The listing builds one solid part. Answer for the finished solid, in the listing's coordinates (mm). Face numbers are marked on the shaded views. A direction names the side the tool comes from. Round coordinates to 2 decimals unless told otherwise and drop trailing zeros. Write each loop counter-clockwise with the first axis right and the second up, starting at its lowest first coordinate (ties: lowest second). Pieces come first, ordered by that corner, then holes. Notation, with made-up numbers: (33.5, -35.5) - (63.5, -35.5) arc R30 ccw to (63.5, 3.5) - close; hole circle Ø4 at (2, 79). An arc over 180 degrees is marked (long way). Use a Markdown table: item, result. Add a question column.
1) A cutting plane is placed at B-B (y = 51.5). Give the vertices of the cut face in (x, z).
2) Find the intervals of material crossed by probe 1 along X at (y, z) = (34.55, 22.5); probe 2 along Y at (x, z) = (63.9, 22.25); probe 3 along Y at (x, z) = (16, 24), in increasing order. Write a range as from..to.
3) Determine the mould class of the marked faces 4, 5 and 6 for opening direction Y: +Y half, -Y half, draft (parallel to the pull), parting line (faces both ways), or undercut.
4) A cutting plane is placed at D-D (y = 43). Give the vertices of the cut face in (x, z), then the cut area to 3 significant figures.
5) A tool of negligible diameter and unlimited length cuts with its end or side. For the marked faces 1, 2 and 3, from which of +Z, -Z, +X, -X, +Y, -Y can it reach the whole face along a straight path? Write none if from no direction.
6) A cutting plane is placed at C-C (x = 71.5). Give the vertices of the cut face in (y, z).
7) A cutting plane is placed at A-A (z = 29.5). Give the vertices of the cut face in (x, y), then the cut area to 3 significant figures.
8) Each of these flat-tipped pins is pushed along its axis until it touches: P1, Ø1.5, axis at x = 42, y = 30.5, coming from the +Z side; P2, Ø1.7, axis at y = 23.5, z = 25.5, coming from the -X side; P3, Ø6, axis at y = 32.5, z = 7.5, coming from the -X side; P4, Ø1.6, axis at x = 16, y = 34.5, coming from the +Z side. Where does it stop, or does it pass through?
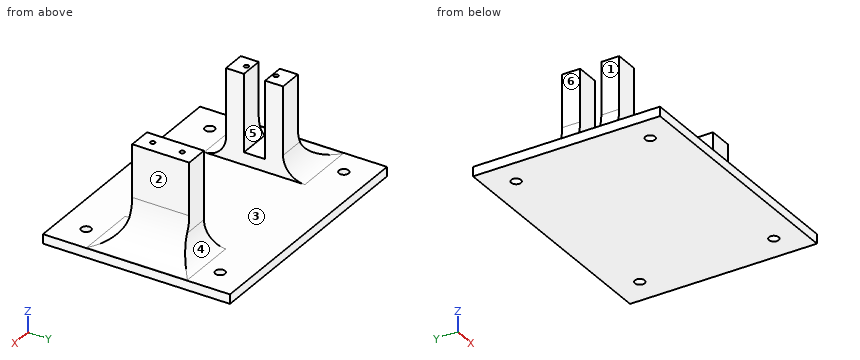
```python
from build123d import *

# Parameters (mm, degrees)
SKETCH078_W     = 80
SKETCH078_H     = 60
PAD029_DEPTH    = 3
SKETCH079_W     = 7.5
SKETCH079_H     = 18.3
PAD030_DEPTH    = 28.8
SKETCH080_R     = 1.55
POCKET038_DEPTH = 5
SKETCH081_R     = 0.75
POCKET039_DEPTH = 15
FILLET024_R     = 12
FILLET025_R     = 7
SKETCH082_W     = 19.5
SKETCH082_H     = 6.8
POCKET040_DEPTH = 24.8


with BuildPart() as part:
    # Sketch078 → Pad029 (new body)
    with BuildSketch(Plane.XY):
        with Locations((40, 30)):
            Rectangle(SKETCH078_W, SKETCH078_H)
    extrude(amount=PAD029_DEPTH)

    # Sketch079 (on Face6 of Pad029) → Pad030 (join)
    with BuildSketch(Plane.XY.offset(3)):
        with Locations((16.1, 30)):
            Rectangle(SKETCH079_W, SKETCH079_H)
        with Locations((63.9, 30)):
            Rectangle(SKETCH079_W, SKETCH079_H)
    extrude(amount=PAD030_DEPTH)

    # Sketch080 (on Face5 of Pad030) → Pocket038 (cut)
    with BuildSketch(Plane.XY.offset(3)):
        with Locations((71.5, 51.5)):
            Circle(SKETCH080_R)
        with Locations((8.5, 51.5)):
            Circle(SKETCH080_R)
        with Locations((71.5, 8.5)):
            Circle(SKETCH080_R)
        with Locations((8.5, 8.5)):
            Circle(SKETCH080_R)
    extrude(amount=-POCKET038_DEPTH, mode=Mode.SUBTRACT)

    # Sketch081 (on Face19 of Pocket038) → Pocket039 (cut)
    with BuildSketch(Plane.XY.offset(31.8)):
        with Locations((16.1, 34.55)):
            Circle(SKETCH081_R)
        with Locations((16.1, 25.05)):
            Circle(SKETCH081_R)
        with Locations((63.9, 34.55)):
            Circle(SKETCH081_R)
        with Locations((63.9, 25.05)):
            Circle(SKETCH081_R)
    extrude(amount=-POCKET039_DEPTH, mode=Mode.SUBTRACT)

    # Fillet024
    fillet024_edges = [part.edges().sort_by_distance(p)[0] for p in [
        (12.35, 30, 3),
        (67.65, 30, 3),
    ]]
    fillet(fillet024_edges, radius=FILLET024_R)

    # Fillet025
    fillet025_edges = [part.edges().sort_by_distance(p)[0] for p in [
        (16.1, 20.85, 3),
        (63.9, 20.85, 3),
        (63.9, 39.15, 3),
        (16.1, 39.15, 3),
    ]]
    fillet(fillet025_edges, radius=FILLET025_R)

    # Sketch082 (on Face19 of Pocket039) → Pocket040 (cut)
    with BuildSketch(Plane.XY.offset(31.8)):
        with Locations((10.1, 30)):
            Rectangle(SKETCH082_W, SKETCH082_H)
    extrude(amount=-POCKET040_DEPTH, mode=Mode.SUBTRACT)


solid = part.part
```
Entries:
| question | item | result |
|---|---|---|
| 1 | outline | (0, 0) - (6.95, 0) - (6.95, 3) - (0, 3) - close; (10.05, 0) - (69.95, 0) - (69.95, 3) - (10.05, 3) - close; (73.05, 0) - (80, 0) - (80, 3) - (73.05, 3) - close |
| 2 | probe 1 | x = 12.35..15.35, 16.85..19.85, 60.15..63.15, 64.65..67.65 |
| 2 | probe 2 | y = 20.85..24.3, 25.8..33.8, 35.3..39.15 |
| 2 | probe 3 | y = 20.85..24.31, 25.79..26.6, 33.4..33.81, 35.29..39.15 |
| 3 | face 4 | +Y half |
| 3 | face 5 | undercut |
| 3 | face 6 | draft |
| 4 | outline | (0, 0) - (80, 0) - (80, 3) - (79.65, 3) arc R12 cw to (75.48, 3.75) - (60.15, 3.75) - (60.15, 3) - (19.85, 3) - (19.85, 3.75) - (4.52, 3.75) arc R12 cw to (0.35, 3) - (0, 3) - close |
| 4 | area | 265 mm² |
| 5 | face 1 | +Z, -X, +Y, -Y |
| 5 | face 2 | +Z, +X, +Y, -Y |
| 5 | face 3 | +Z |
| 6 | outline | (0, 0) - (6.95, 0) - (6.95, 3) - (0, 3) - close; (10.05, 0) - (49.95, 0) - (49.95, 3) - (46.15, 3) arc R7 cw to (40.28, 6.19) - (19.72, 6.19) arc R7 cw to (13.85, 3) - (10.05, 3) - close; (53.05, 0) - (60, 0) - (60, 3) - (53.05, 3) - close |
| 7 | outline | (12.35, 20.85) - (19.85, 20.85) - (19.85, 26.6) - (12.35, 26.6) - close; (12.35, 33.4) - (19.85, 33.4) - (19.85, 39.15) - (12.35, 39.15) - close; (60.15, 20.85) - (67.65, 20.85) - (67.65, 39.15) - (60.15, 39.15) - close; hole circle Ø1.5 at (16.1, 25.05); hole circle Ø1.5 at (16.1, 34.55); hole circle Ø1.5 at (63.9, 25.05); hole circle Ø1.5 at (63.9, 34.55) |
| 7 | area | 216 mm² |
| 8 | P1 | stops at z = 3 |
| 8 | P2 | stops at x = 12.35 |
| 8 | P3 | stops at x = 6.16 |
| 8 | P4 | stops at z = 31.8 |
